Can you work these out from the model? Positions are in its coordinate system, mm. Face numbers are marked on the shaded views. A direction names the side the tool comes from. Coordinates: 2 decimals unless noted, no trailing zeros. Order: outer loops, then holes, each group sorted by start corner. A loop starts at its lowest first (then second) coordinate and runs counter-clockwise, first axis right, second up. Notation, with made-up numbers: (17.25, 5) -> (29.25, 5) arc R29 cw to (29.25, 43) -> close; hole circle Ø9 at (13, 5.5). An arc over 180 degrees is marked (long way). Use a Markdown table: item, result. Add a question column.
1. Suppose I cut it at A-A, the plane z = -1.5. List the corners of the cut face in (x, y) for me, then the cut area to 3 significant figures.
2. Suppose I cut it at C-C, the plane x = 250.5. List the corners of the cut face in (y, z) for me, then the cut area to 3 significant figures.
3. For pin 1 Ø8 at (x, z) = (194, -8) entering from -Y; pin 2 Ø4 at (x, z) = (139.5, 2.5) entering from +Y; pin 3 Ø12 at (x, z) = (110.5, -8) entering from +Y; pin 4 Ø4 at (x, y) = (62.51, 43.16) entering from -Z, each with a flat end and sliding along its axis, tell me the tip position at first contact or that it passes through.
4. If I drill on line 1 along Z through (x, y) = (270.5, 97); line 2 along X through (y, z) = (43.5, -2.25); line 3 along X through (y, z) = (102, 7.5), over which ranges is the centre line in solid material (lowest first)? Write a range as from..to.
5. For the marked faces 1 and 2, which set-ups out of +Z, -Z, +X, -X, +Y, -Y let a thin tool reach every point of the face, with its end or its side?
6. Suppose I cut it at B-B, the plane y = 66. List the corners of the cut face in (x, z) for me, then the cut area to 3 significant figures.
```python
from build123d import *

# Parameters (mm, degrees)
EXTRUDE_1_DEPTH          = 7
EXTRUDE_1_DEPTH_BACK     = 7
SKETCH_1_R               = 1.5
FILLET_1_R               = 10
EXTRUDE_2_DEPTH          = 2.9
EXTRUDE_2_DEPTH_BACK     = 2.8
SKETCH_3_R               = 1.5
CUT_EXTRUDE_1_DEPTH      = 5.2
CUT_EXTRUDE_1_DEPTH_BACK = 5.2
SCALE1_SCALE             = 1.5


with BuildPart() as part:
    # Sketch 1 → Extrude 1 (new, two sides: drawn at the far end of the back side and taken through both)
    with BuildSketch(Plane.XY.offset(-EXTRUDE_1_DEPTH_BACK)):
        with BuildLine():
            ThreePointArc((240.699236038, 105.645995337), (243.6, 101.8), (240.699236038, 97.954004663))
            Line((240.699236038, 97.954004663), (232.071936087, 95.488208898))
            Line((232.071936087, 95.488208898), (163.6, 91.5))
            ThreePointArc((163.6, 91.5), (147.125308547, 88.283437456), (132.1, 80.8))
            Line((132.1, 80.8), (97.347754748, 57.19128445))
            ThreePointArc((97.347754748, 57.19128445), (92.03920173, 57.924827394), (92.224555949, 63.280615311))
            Line((92.224555949, 63.280615311), (128.7, 101))
            ThreePointArc((128.7, 101), (143.303490983, 110.55954938), (160.6, 112.9))
            Line((160.6, 112.9), (232.071936087, 108.111791102))
            Line((232.071936087, 108.111791102), (240.699236038, 105.645995337))
        make_face()
        with Locations((95.1, 60.5)):
            Circle(SKETCH_1_R, mode=Mode.SUBTRACT)
        with Locations((152.6, 99.603139307)):
            Circle(SKETCH_1_R, mode=Mode.SUBTRACT)
        with Locations((239.6, 101.8)):
            Circle(SKETCH_1_R, mode=Mode.SUBTRACT)
    extrude(amount=EXTRUDE_1_DEPTH + EXTRUDE_1_DEPTH_BACK)

    # Fillet 1
    fillet_1_edges = [part.edges().sort_by_distance(p)[0] for p in [
        (232.071936087, 95.488208898, 0),
        (232.071936087, 108.111791102, 0),
    ]]
    fillet(fillet_1_edges, radius=FILLET_1_R)

    # Sketch 3 → Extrude 2 (add, two sides: drawn at the far end of the back side and taken through both)
    with BuildSketch(Plane.XY.offset(-EXTRUDE_2_DEPTH_BACK)):
        with BuildLine():
            Line((160.6, 112.9), (163.651401787, 112.69557362))
            Line((163.651401787, 112.69557362), (163.893737551, 116.312835642))
            ThreePointArc((163.893737551, 116.312835642), (162.654460758, 118.828873494), (159.855517856, 119.008239262))
            Line((159.855517856, 119.008239262), (139.549521827, 108.933263618))
            ThreePointArc((139.549521827, 108.933263618), (149.801009446, 112.369362402), (160.6, 112.9))
        make_face()
        with Locations((161.1, 116.5)):
            Circle(SKETCH_3_R, mode=Mode.SUBTRACT)
    extrude(amount=EXTRUDE_2_DEPTH + EXTRUDE_2_DEPTH_BACK)

    # Sketch 4 → Cut-Extrude 1 (cut, two sides: drawn at the far end of the back side and taken through both)
    with BuildSketch(Plane.XY.offset(-CUT_EXTRUDE_1_DEPTH_BACK)):
        with BuildLine():
            Line((231.012866709, 108.182742662), (224.6, 108.612367871))
            Line((224.6, 108.612367871), (228.236474469, 103.550312019))
            ThreePointArc((228.236474469, 103.550312019), (228.799985675, 101.790729145), (228.225610058, 100.034662683))
            Line((228.225610058, 100.034662683), (224.6, 95.052999327))
            Line((224.6, 95.052999327), (230.968280992, 95.423925524))
            ThreePointArc((230.968280992, 95.423925524), (232.061731819, 95.548272011), (233.134897693, 95.792017302))
            Line((233.134897693, 95.792017302), (240.699236038, 97.954004663))
            ThreePointArc((240.699236038, 97.954004663), (243.6, 101.8), (240.699236038, 105.645995337))
            Line((240.699236038, 105.645995337), (233.092512669, 107.820096895))
            ThreePointArc((233.092512669, 107.820096895), (232.062285935, 108.056450871), (231.012866709, 108.182742662))
        make_face()
    extrude(amount=CUT_EXTRUDE_1_DEPTH + CUT_EXTRUDE_1_DEPTH_BACK, mode=Mode.SUBTRACT)


with BuildPart() as part_1:
    # Scale1: scaled about (160.287784575, 95.185568028, 0.00047642)
    add(part.part.scale(SCALE1_SCALE).moved(Location((-80.143892287, -47.592784014, -0.00023821))))


solid = part_1.part
```
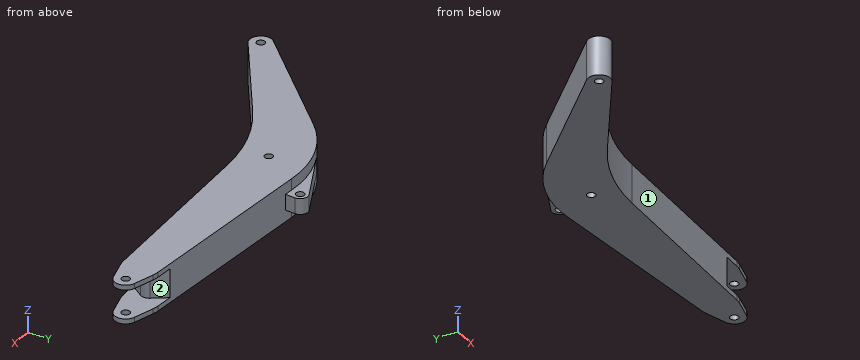
Worked out:
| question | item | result |
|---|---|---|
| 1 | outline | (58.19, 47.33) arc R6 ccw to (65.88, 38.19) -> (118.01, 73.61) arc R93.79 cw to (165.26, 89.66) -> (256.76, 94.99) -> (262.19, 102.46) arc R4.5 ccw to (262.21, 107.73) -> (256.76, 115.33) -> (165.33, 121.45) -> (165.7, 126.88) arc R4.2 ccw to (159.64, 130.92) -> (129.18, 115.81) arc R59.31 ccw to (112.91, 103.91) -> close; hole circle Ø4.5 at (62.51, 43.16); hole circle Ø4.5 at (148.76, 101.81); hole circle Ø4.5 at (161.51, 127.16) |
| 1 | area | 5,680 mm² |
| 2 | outline | (94.62, -10.5) -> (115.74, -10.5) -> (115.74, 10.5) -> (94.62, 10.5) -> close |
| 2 | area | 444 mm² |
| 3 | pin 1 | stops at y = 91.1 |
| 3 | pin 2 | stops at y = 121.92 |
| 3 | pin 3 | stops at y = 107.33 |
| 3 | pin 4 | passes through |
| 4 | line 1 | z = -10.5..-7.8, 7.8..10.5 |
| 4 | line 2 | x = 56.52..60.28, 64.73..73.69 |
| 4 | line 3 | x = 111.06..146.51, 151..261.86 |
| 5 | face 1 | +Z, -Z, +X, -Y |
| 5 | face 2 | +X, +Y |
| 6 | outline | (76.25, -10.5) -> (106.81, -10.5) -> (106.81, 10.5) -> (76.25, 10.5) -> close |
| 6 | area | 642 mm² |
